Autodesk Inventor part; units mm, degrees
ref_plane "YZ Plane" through (0, 0, 0) normal (1, 0, 0) x (0, 1, 0)
ref_plane "XZ Plane" through (0, 0, 0) normal (0, 1, 0) x (-1, 0, 0)
ref_plane "XY Plane" through (0, 0, 0) normal (0, 0, 1) x (1, 0, 0)
sketch "スケッチ1" plane through (0, 0, 0) normal (1, 0, 0) x (0, 1, 0)
  circle A0 centre (0, 0) radius 3
  circle A1 centre (0, 0) radius 5 construction
  arc A2 (6.9378, -3.9834) -> (-6.9378, -3.9834) centre (0, 0) ccw
  arc A3 (6.9378, -3.9834) -> (4.0719, -16.7819) centre (26.125, -15) ccw
  arc A4 (-4.0719, -16.7819) -> (-6.9378, -3.9834) centre (-26.125, -15) ccw
  arc A5 (4.0719, -16.7819) -> (7.5605, -20) centre (7.5605, -16.5) ccw
  arc A6 (-7.5605, -20) -> (-4.0719, -16.7819) centre (-7.5605, -16.5) ccw
  line L0 (7.5605, -20) -> (17.5, -20)
  line L1 (20.2879, -21.384) -> (25.5362, -28.299)
  line L2 (17, -32.909) -> (17, -27)
  line L3 (16, -26) -> (-16, -26)
  line L4 (-17, -27) -> (-17, -32.909)
  line L5 (-25.5362, -28.299) -> (-20.2879, -21.384)
  line L6 (-17.5, -20) -> (-7.5605, -20)
  arc A7 (-25.2033, -31.0612) -> (-20, -34.641) centre (0, 0) ccw
  arc A8 (20, -34.641) -> (25.2033, -31.0612) centre (0, 0) ccw
  arc A9 (25.2033, -31.0612) -> (25.5362, -28.299) centre (23.9431, -29.5081) ccw
  arc A10 (17, -32.909) -> (20, -34.641) centre (19, -32.909) ccw
  arc A11 (-20, -34.641) -> (-17, -32.909) centre (-19, -32.909) ccw
  arc A12 (-25.5362, -28.299) -> (-25.2033, -31.0612) centre (-23.9431, -29.5081) ccw
  arc A13 (-17.5, -20) -> (-20.2879, -21.384) centre (-17.5, -23.5) ccw
  arc A14 (20.2879, -21.384) -> (17.5, -20) centre (17.5, -23.5) ccw
  line L7 (0, 0) -> (0, -40) construction
  arc A15 (-20, -34.641) -> (20, -34.641) centre (0, 0) ccw construction
  arc A16 (17, -27) -> (16, -26) centre (16, -27) ccw
  arc A17 (-16, -26) -> (-17, -27) centre (-16, -27) ccw
  line L8 (4, 0) -> (4, -38.6169) construction
  line L9 (26.125, -15) -> (-26.125, -15) construction
  point P0 (26.6783, -29.8038)
  point P1 (17, -36.2077)
  point P2 (-17, -36.2077)
  point P3 (-26.6783, -29.8038)
  dimension "d0" = 10
  dimension "d1" = 2
  dimension "d2" = 3.5
  dimension "d4" = 1
  dimension "d5" = 8
  dimension "d6" = 6
  dimension "d7" = 8
  dimension "d8" = 26
  dimension "d9" = 6
  dimension "d10" = 6
  dimension "d11" = 34
  dimension "d12" = 15
  dimension "d13" = 35
  dimension "d16" = 14
extrude "押し出し1" add sketch "スケッチ1" along normal blind 2
properties part number "camera_stay"
For this review, take the finished solid that the model builds, in its own axes (mm). A direction names the side the tool comes from. Round coordinates to 2 decimals unless told otherwise and drop trailing zeros. Write each loop counter-clockwise with the first axis right and the second up, starting at its lowest first coordinate (ties: lowest second). Pieces come first, ordered by that corner, then holes.
1) Insertion check: pin 1 Ø6 at (y, z) = (9.5, -7.5) entering from +X; pin 2 Ø1 at (x, y) = (1.5, -16) entering from -Z; pin 3 Ø1 at (x, y) = (1, -6.5) entering from -Z; pin 4 Ø1 at (x, y) = (1, 12.5) entering from +Z. Each pin has a flat end and moves straight along its axis. Give the tip position at first contact, or say it passes through.
Answer below:
pin 1: passes through
pin 2: stops at z = -26.13
pin 3: stops at z = -26
pin 4: stops at z = -20
2) Take a section at D-D on y = 13.5. Give the boundary of the cut face in (x, z).
Answer below:
outline: (0, -26) - (2, -26) - (2, -20) - (0, -20) - close
3) Take a section at A-A on z = 0. Give the boundary of the cut face in (x, y).
Answer below:
outline: (0, -8) - (2, -8) - (2, -3) - (0, -3) - close; (0, 3) - (2, 3) - (2, 8) - (0, 8) - close
4) Machinability: for faces 4 (the face through (0.986, 5.214, -19.097)), 5 (the face through (1, -17, -30)), 6 (the face through (2, 0, -17)), 7 (the face through (0.986, 19.036, -20.355)), 8 (the face through (0.986, -5.161, -19.048)), which of the approach directions +Z, -Z, +X, -X, +Y, -Y give a long, thin tool a straight path to every point of the face, cutting with its end or side? Answer none if there is none.
Answer below:
face 4: +X, -X, +Y
face 5: -Z, +X, -X
face 6: +Z, -Z, +X, +Y, -Y
face 7: +Z, +X, -X, +Y
face 8: +X, -X, -Y
5) Take a section at B-B on y = 0. Give the boundary of the cut face in (x, z).
Answer below:
outline: (0, -26) - (2, -26) - (2, -3) - (0, -3) - close; (0, 3) - (2, 3) - (2, 8) - (0, 8) - close
6) Mouldability with a two-part tool opening along Y and no side actions: class faces 1 (the face through (1, 0, -26)), 2 (the face through (0.986, -25.926, -29.769)), 3 (the face through (1, -13, -20)) as +Y half, -Y half, draft (parallel to the pull), parting line (faces both ways), or undercut.
Answer below:
face 1: undercut
face 2: -Y half
face 3: draft
7) For line 1 along Z through (x, y) = (0.95, 0); line 2 along Z through (x, y) = (1.8, -14.5); line 3 along Y through (x, z) = (1.55, -4), list the stretches that pass through material, from the lowest coordinate up.
Answer below:
line 1: z = -26 to -3, 3 to 8
line 2: z = -26 to -20
line 3: y = -6.93 to 6.93
8) Take a section at C-C on x = 0.3. Give the boundary of the cut face in (y, z), then the cut area to 3 significant figures.
Answer below:
outline: (-25.54, -28.3) arc R2 ccw to (-25.2, -31.06) arc R39.99 ccw to (-20, -34.64) arc R2 ccw to (-17, -32.91) - (-17, -27) arc R1 cw to (-16, -26) - (16, -26) arc R1 cw to (17, -27) - (17, -32.91) arc R2 ccw to (20, -34.64) arc R40.01 ccw to (25.2, -31.06) arc R2 ccw to (25.54, -28.3) - (20.29, -21.38) arc R3.5 ccw to (17.5, -20) - (7.56, -20) arc R3.5 cw to (4.07, -16.78) arc R22.13 cw to (6.94, -3.98) arc R8 ccw (long way) to (-6.94, -3.98) arc R22.12 cw to (-4.07, -16.78) arc R3.5 cw to (-7.56, -20) - (-17.5, -20) arc R3.5 ccw to (-20.29, -21.38) - close; hole circle Ø6 at (0, 0)
area: 670 mm2
